Autodesk Fusion 360 part; units mm, degrees
sketch "wheel" plane through (0, 0, 0) normal (0, 0, 1) x (1, 0, 0)
  circle A0 centre (0, 0) radius 19.05
  line L0 (-3.1964, 18.7799) -> (-3.1964, 22.86)
  line L1 (-3.1964, 22.86) -> (3.1964, 22.86)
  line L2 (3.1964, 22.86) -> (3.1964, 18.7799)
  line L3 (-13.6245, 13.3144) -> (-16.0227, 16.6153)
  line L4 (-16.0227, 16.6153) -> (-10.8508, 20.3729)
  line L5 (-10.8508, 20.3729) -> (-8.4526, 17.0721)
  line L6 (-18.8485, 2.7633) -> (-22.7289, 4.0241)
  line L7 (-22.7289, 4.0241) -> (-20.7534, 10.1041)
  line L8 (-20.7534, 10.1041) -> (-16.873, 8.8433)
  line L9 (-16.873, -8.8433) -> (-20.7534, -10.1041)
  line L10 (-20.7534, -10.1041) -> (-22.7289, -4.0241)
  line L11 (-22.7289, -4.0241) -> (-18.8485, -2.7633)
  line L12 (-8.4526, -17.0721) -> (-10.8508, -20.373)
  line L13 (-10.8508, -20.373) -> (-16.0227, -16.6153)
  line L14 (-16.0227, -16.6153) -> (-13.6245, -13.3145)
  line L15 (3.1964, -18.7799) -> (3.1964, -22.86)
  line L16 (3.1964, -22.86) -> (-3.1964, -22.86)
  line L17 (-3.1964, -22.86) -> (-3.1964, -18.7799)
  line L18 (13.6245, -13.3144) -> (16.0227, -16.6153)
  line L19 (16.0227, -16.6153) -> (10.8508, -20.3729)
  line L20 (10.8508, -20.3729) -> (8.4526, -17.0721)
  line L21 (18.8485, -2.7633) -> (22.7289, -4.0241)
  line L22 (22.7289, -4.0241) -> (20.7534, -10.1041)
  line L23 (20.7534, -10.1041) -> (16.873, -8.8433)
  line L24 (16.873, 8.8433) -> (20.7534, 10.1041)
  line L25 (20.7534, 10.1041) -> (22.7289, 4.0241)
  line L26 (22.7289, 4.0241) -> (18.8485, 2.7633)
  line L27 (8.4526, 17.0721) -> (10.8508, 20.373)
  line L28 (10.8508, 20.373) -> (16.0227, 16.6153)
  line L29 (16.0227, 16.6153) -> (13.6245, 13.3145)
  dimension "d1" = 38.1
  dimension "d2" = 6.3929
  dimension "d3" = 4.0801
  dimension "d5" = 360
extrude "Extrude1" add sketch "wheel" along normal blind 3.81
sketch "hole punch" plane through (0, 0, 3.81) normal (0, 0, 1) x (-1, 0, 0)
  arc A0 (-8.4526, -17.0721) -> (-3.1964, -18.7799) centre (0, 0) ccw
  line L0 (-3.1964, -18.7799) -> (-3.1964, -22.86)
  line L1 (-3.1964, -22.86) -> (3.1964, -22.86)
  line L2 (3.1964, -22.86) -> (3.1964, -18.7799)
  arc A1 (3.1964, -18.7799) -> (8.4526, -17.0721) centre (0, 0) ccw
  line L3 (8.4526, -17.0721) -> (10.8508, -20.3729)
  line L4 (10.8508, -20.3729) -> (16.0227, -16.6153)
  line L5 (16.0227, -16.6153) -> (13.6245, -13.3144)
  arc A2 (13.6245, -13.3144) -> (16.873, -8.8433) centre (0, 0) ccw
  line L6 (16.873, -8.8433) -> (20.7534, -10.1041)
  line L7 (20.7534, -10.1041) -> (22.7289, -4.0241)
  line L8 (22.7289, -4.0241) -> (18.8485, -2.7633)
  arc A3 (18.8485, -2.7633) -> (18.8485, 2.7633) centre (0, 0) ccw
  line L9 (18.8485, 2.7633) -> (22.7289, 4.0241)
  line L10 (22.7289, 4.0241) -> (20.7534, 10.1041)
  line L11 (20.7534, 10.1041) -> (16.873, 8.8433)
  arc A4 (16.873, 8.8433) -> (13.6245, 13.3145) centre (0, 0) ccw
  line L12 (13.6245, 13.3145) -> (16.0227, 16.6153)
  line L13 (16.0227, 16.6153) -> (10.8508, 20.373)
  line L14 (10.8508, 20.373) -> (8.4526, 17.0721)
  arc A5 (8.4526, 17.0721) -> (3.1964, 18.7799) centre (0, 0) ccw
  line L15 (3.1964, 18.7799) -> (3.1964, 22.86)
  line L16 (3.1964, 22.86) -> (-3.1964, 22.86)
  line L17 (-3.1964, 22.86) -> (-3.1964, 18.7799)
  arc A6 (-3.1964, 18.7799) -> (-8.4526, 17.0721) centre (0, 0) ccw
  line L18 (-8.4526, 17.0721) -> (-10.8508, 20.3729)
  line L19 (-10.8508, 20.3729) -> (-16.0227, 16.6153)
  line L20 (-16.0227, 16.6153) -> (-13.6245, 13.3144)
  arc A7 (-13.6245, 13.3144) -> (-16.873, 8.8433) centre (0, 0) ccw
  line L21 (-16.873, 8.8433) -> (-20.7534, 10.1041)
  line L22 (-20.7534, 10.1041) -> (-22.7289, 4.0241)
  line L23 (-22.7289, 4.0241) -> (-18.8485, 2.7633)
  arc A8 (-18.8485, 2.7633) -> (-18.8485, -2.7633) centre (0, 0) ccw
  line L24 (-18.8485, -2.7633) -> (-22.7289, -4.0241)
  line L25 (-22.7289, -4.0241) -> (-20.7534, -10.1041)
  line L26 (-20.7534, -10.1041) -> (-16.873, -8.8433)
  arc A9 (-16.873, -8.8433) -> (-13.6245, -13.3145) centre (0, 0) ccw
  line L27 (-13.6245, -13.3145) -> (-16.0227, -16.6153)
  line L28 (-16.0227, -16.6153) -> (-10.8508, -20.373)
  line L29 (-10.8508, -20.373) -> (-8.4526, -17.0721)
  circle A10 centre (0, 0) radius 19.05
  line L30 (0.0528, -19.0499) -> (0.0528, 19.0499)
  line L31 (19.05, 0) -> (-19.05, 0)
hole "Hole1" at (0, 0, 3.81) direction (0, 0, -1) diameter 6.2 depth 6.2 tip angle 118
The listing builds one solid part. Answer for the finished solid, in the listing's coordinates (mm). A direction names the side the tool comes from. Give positions to 0.01 mm unless a question says otherwise; leave off trailing zeros. Order: outer loops, then holes, each group sorted by start corner. A loop starts at its lowest first (then second) coordinate and runs counter-clockwise, first axis right, second up. Notation, with made-up numbers: (2, -33.5) -> (16, -33.5) arc R18 cw to (16, -24.5) -> close; hole circle Ø11 at (-21, 27). An arc over 180 degrees is marked (long way). One line per item, written item: value.
1) Flat-ended cylindrical pins translate along their axes: P1, Ø1, axis at y = -6.5, z = 2.5, coming from the -X side; P2, Ø2, axis at x = 9.5, z = 2, coming from the +Y side; P3, Ø1.9, axis at y = -20.5, z = 1.5, coming from the +X side. Find the tip coordinate at first contact, or state that the pin passes through.
Reported:
P1: stops at x = -22.09
P2: stops at y = 19.89
P3: stops at x = 11.98
2) A tool of negligible diameter and unlimited length cuts with its end or side. For faces 1 (the flat face through (20.762, -3.385, 1.878)), 2 (the cylindrical face through (5.85, 18.13, 1.88)), 3 (the flat face through (3.196, -21, 2)), 4 (the flat face through (-14.84, -14.99, 1.88)), from which of +Z, -Z, +X, -X, +Y, -Y can it reach the whole face along a straight path? Write none if from no direction.
Reported:
face 1: +Z, -Z, +X
face 2: +Z, -Z, +Y
face 3: +Z, -Z, -Y
face 4: +Z, -Z, -X
3) Find section D-D, the plane x = -18. Determine the outline of the cut face in (y, z).
Reported:
outline: (-9.21, 0) -> (9.21, 0) -> (9.21, 3.81) -> (-9.21, 3.81) -> close
4) Find section B-B, the plane y = 0. Determine the outline of the cut face in (x, z), plus the area to 3 significant figures.
Reported:
outline: (-19.05, 0) -> (-3.1, 0) -> (-3.1, 3.81) -> (-19.05, 3.81) -> close; (3.1, 0) -> (19.05, 0) -> (19.05, 3.81) -> (3.1, 3.81) -> close
area: 122 mm^2
5) Find the intervals of material crossed by line 1 (Y direction, x = 0, z = 2.9); line 2 (X direction, y = 0, z = 1.3); line 3 (Y direction, x = 14, z = 1), in increasing order.
Reported:
line 1: y = -22.86 to -3.1, 3.1 to 22.86
line 2: x = -19.05 to -3.1, 3.1 to 19.05
line 3: y = -18.08 to -13.83, -12.92 to 12.92, 13.83 to 18.08
6) Determine the mould class of faces 5 (the flat face through (-20.816, -3.403, 1.878)), 6 (the flat face through (-3.196, -21, 2)), 7 (the flat face through (0, 22.86, 2)) for opening direction X: pulls with the +X half, pulls with the -X half, needs draft (parallel to the pull), parting line crosses it, or undercut.
Reported:
face 5: pulls with the -X half
face 6: undercut
face 7: needs draft
7) Find section A-A, the plane x = 0. Determine the outline of the cut face in (y, z).
Reported:
outline: (-22.86, 0) -> (-3.1, 0) -> (-3.1, 3.81) -> (-22.86, 3.81) -> close; (3.1, 0) -> (22.86, 0) -> (22.86, 3.81) -> (3.1, 3.81) -> close
8) Find section C-C, the plane y = 15.5. Determine the outline of the cut face in (x, z), plus the area to 3 significant figures.
Reported:
outline: (-15.21, 0) -> (15.21, 0) -> (15.21, 3.81) -> (-15.21, 3.81) -> close
area: 116 mm^2
